For this review, take the finished solid that the model builds, in its own axes (mm). Face numbers are marked on the shaded views. Round coordinates to 2 decimals unless told otherwise and drop trailing zeros. Loops run counter-clockwise (first coordinate to the right, second up) from the corner with the lowest first, then second, coordinate; pieces in that order, holes last.
1. Clearance check with flat-ended pins moving along their axes: pin 1 Ø7.5 at (x, y) = (-84.5, 78.5) entering from +Z; pin 2 Ø2.5 at (y, z) = (-84.5, 11) entering from +X; pin 3 Ø4 at (x, z) = (-86.5, 10) entering from -Y. State where each tip first meets the part, or that it passes through.
2. Draft analysis for pull direction Y (two halves, no side actions). For the marked faces 1, 2, 3 and 4, state which applies: released by +Y, released by -Y, zero draft, split by the parting line, or undercut.
3. To check wall thickness, follow line 1 along Y through (x, z) = (-79.2, 12); line 2 along Y through (x, z) = (45, 9.5). State the ranges of each line that lie inside material, in increasing order.
4. Consider section A-A on x = -7.5. State the section outline as (y, z) points, then the cut area to 3 significant figures.
5. Consider section C-C on y = 85. State the section outline as (x, z) points, then the cut area to 3 significant figures.
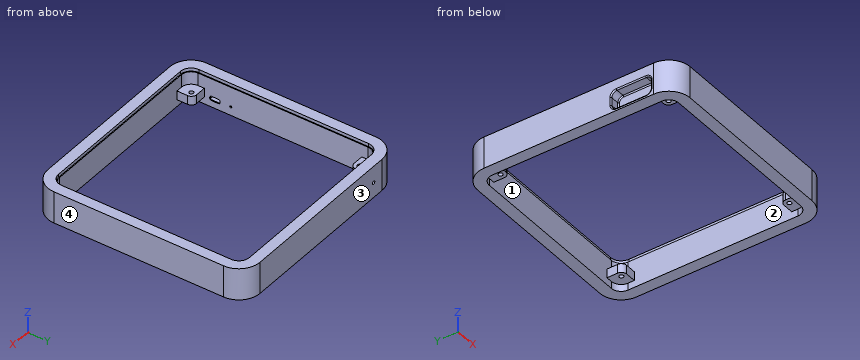
from build123d import *

# Parameters (mm, degrees)
SKETCH2_W                = 200
SKETCH2_H                = 200
BOSS_EXTRUDE1_DEPTH      = 30
FILLET1_R                = 20
CUT_EXTRUDE1_DEPTH       = 3
CUT_EXTRUDE2_DEPTH       = 28
SKETCH6_W                = 15
SKETCH6_H                = 15
BOSS_EXTRUDE4_DEPTH      = 15
FILLET2_R                = 5
F_4_0_4_DIAMETER_HOLE1_D = 4
CUT_EXTRUDE3_DEPTH       = 6.6
CUT_EXTRUDE4_REACH       = 202
SKETCH11_R               = 1.5
SKETCH15_R               = 1
CUT_EXTRUDE5_DEPTH       = 11.8
CUT_EXTRUDE7_DEPTH       = 9.8
FILLET3_R                = 1


with BuildPart() as part:
    # Sketch2 → Boss-Extrude1 (new body)
    with BuildSketch(Plane.XY):
        Rectangle(SKETCH2_W, SKETCH2_H)
    extrude(amount=BOSS_EXTRUDE1_DEPTH)

    # Fillet1
    fillet1_edges = [part.edges().sort_by_distance(p)[0] for p in [
        (100, -100, 15),
        (-100, -100, 15),
        (-100, 100, 15),
        (100, 100, 15),
    ]]
    fillet(fillet1_edges, radius=FILLET1_R)

    # Sketch3 → Cut-Extrude1 (cut)
    with BuildSketch(Plane.XY.offset(30)):
        with BuildLine():
            Line((-90, 80), (-90, -80))
            ThreePointArc((-90, -80), (-87.071067812, -87.071067812), (-80, -90))
            Line((-80, -90), (80, -90))
            ThreePointArc((80, -90), (87.071067812, -87.071067812), (90, -80))
            Line((90, -80), (90, 80))
            ThreePointArc((90, 80), (87.071067812, 87.071067812), (80, 90))
            Line((80, 90), (-80, 90))
            ThreePointArc((-80, 90), (-87.071067812, 87.071067812), (-90, 80))
        make_face()
    extrude(amount=-CUT_EXTRUDE1_DEPTH, mode=Mode.SUBTRACT)

    # Sketch4 → Cut-Extrude2 (cut, through all)
    with BuildSketch(Plane.XY.offset(27)):
        with BuildLine():
            Line((-89.2, 80), (-89.2, -80))
            ThreePointArc((-89.2, -80), (-86.505382387, -86.505382387), (-80, -89.2))
            Line((-80, -89.2), (80, -89.2))
            ThreePointArc((80, -89.2), (86.505382387, -86.505382387), (89.2, -80))
            Line((89.2, -80), (89.2, 80))
            ThreePointArc((89.2, 80), (86.505382387, 86.505382387), (80, 89.2))
            Line((80, 89.2), (-80, 89.2))
            ThreePointArc((-80, 89.2), (-86.505382387, 86.505382387), (-89.2, 80))
        make_face()
    extrude(amount=-CUT_EXTRUDE2_DEPTH, mode=Mode.SUBTRACT)

    # Sketch6 → Boss-Extrude4 (add)
    with BuildSketch(Plane(origin=(0, 0, 0), x_dir=(-1, 0, 0), z_dir=(0, 0, -1))):
        with Locations((-81.7, -81.7)):
            Rectangle(SKETCH6_W, SKETCH6_H)
        with Locations((-81.7, 81.7)):
            Rectangle(SKETCH6_W, SKETCH6_H)
        with Locations((81.7, 81.7)):
            Rectangle(SKETCH6_W, SKETCH6_H)
        with Locations((81.7, -81.7)):
            Rectangle(SKETCH6_W, SKETCH6_H)
    extrude(amount=-BOSS_EXTRUDE4_DEPTH)

    # Fillet2
    fillet2_edges = [part.edges().sort_by_distance(p)[0] for p in [
        (74.2, 74.2, 7.5),
        (-74.2, 74.2, 7.5),
        (-74.2, -74.2, 7.5),
        (74.2, -74.2, 7.5),
    ]]
    fillet(fillet2_edges, radius=FILLET2_R)

    # Ø4.0 (4) Diameter Hole1 (through all)
    with Locations(Plane(origin=(0, 0, 0), x_dir=(-1, 0, 0), z_dir=(0, 0, -1))):
        with Locations((-79.2, 79.2), (79.2, 79.2), (-79.2, -79.2), (79.2, -79.2)):
            Hole(F_4_0_4_DIAMETER_HOLE1_D / 2)

    # Sketch10 → Cut-Extrude3 (cut)
    with BuildSketch(Plane(origin=(0, 0, 0), x_dir=(-1, 0, 0), z_dir=(0, 0, -1))):
        with BuildLine():
            Line((89.2, -80), (89.2, 80))
            ThreePointArc((89.2, 80), (86.505382387, 86.505382387), (80, 89.2))
            Line((80, 89.2), (-80, 89.2))
            ThreePointArc((-80, 89.2), (-86.505382387, 86.505382387), (-89.2, 80))
            Line((-89.2, 80), (-89.2, -80))
            ThreePointArc((-89.2, -80), (-86.505382387, -86.505382387), (-80, -89.2))
            Line((-80, -89.2), (80, -89.2))
            ThreePointArc((80, -89.2), (86.505382387, -86.505382387), (89.2, -80))
        make_face()
    extrude(amount=-CUT_EXTRUDE3_DEPTH, mode=Mode.SUBTRACT)

    # Sketch11 → Cut-Extrude4 (cut, up to next)
    with BuildSketch(Plane(origin=(0, 100, 0), x_dir=(1, 0, 0), z_dir=(0, 1, 0)), mode=Mode.PRIVATE) as cut_extrude4_sk1:
        with Locations((-68.95500318, -14.324851484)):
            Circle(SKETCH11_R)
    cut_extrude4_tool1 = extrude(cut_extrude4_sk1.sketch, amount=-CUT_EXTRUDE4_REACH, mode=Mode.PRIVATE) & part.part
    add(cut_extrude4_tool1.solids().sort_by_distance((-68.955003, 100, 14.324851))[0], mode=Mode.SUBTRACT)

    # Sketch15 → Cut-Extrude5 (cut, through all)
    with BuildSketch(Plane(origin=(-89.2, 0, 0), x_dir=(0, 0, -1), z_dir=(1, 0, 0))):
        with Locations((-8.179999988, -49.23845191)):
            Circle(SKETCH15_R)
        with BuildLine():
            Line((-6.1, -64.178451904), (-6.1, -64.148451912))
            Line((-6.1, -64.148451912), (-6.1, -60.988451904))
            ThreePointArc((-6.1, -60.988451904), (-6.237016841, -60.299621726), (-6.627207794, -59.715659698))
            ThreePointArc((-6.627207794, -59.715659698), (-7.211170067, -59.325468644), (-7.90000053, -59.188451904))
            Line((-7.90000053, -59.188451904), (-8.46, -59.188451904))
            ThreePointArc((-8.46, -59.188451904), (-9.148830178, -59.325468746), (-9.732792206, -59.715659698))
            ThreePointArc((-9.732792206, -59.715659698), (-10.122983159, -60.299621726), (-10.26, -60.988451904))
            Line((-10.26, -60.988451904), (-10.26, -67.338451904))
            ThreePointArc((-10.26, -67.338451904), (-10.122983159, -68.027282082), (-9.732792205, -68.611244109))
            ThreePointArc((-9.732792205, -68.611244109), (-9.148830178, -69.001435061), (-8.46, -69.138451901))
            Line((-8.46, -69.138451901), (-7.900000051, -69.138451901))
            ThreePointArc((-7.900000051, -69.138451901), (-7.211169847, -69.001435069), (-6.627207798, -68.611244107))
            ThreePointArc((-6.627207798, -68.611244107), (-6.237016846, -68.02728208), (-6.100000002, -67.338451904))
            Line((-6.100000002, -67.338451904), (-6.1, -64.178451904))
        make_face()
    extrude(amount=-CUT_EXTRUDE5_DEPTH, mode=Mode.SUBTRACT)

    # Sketch17 → Cut-Extrude7 (cut)
    with BuildSketch(Plane.ZY.offset(100)):
        with BuildLine():
            Line((15.061316978, -39.847521487), (7.5, -39.847521487))
            ThreePointArc((7.5, -39.847521487), (3.964466094, -41.311987581), (2.5, -44.847521487))
            Line((2.5, -44.847521487), (2.5, -72.5))
            ThreePointArc((2.5, -72.5), (3.964466094, -76.035533906), (7.5, -77.5))
            Line((7.5, -77.5), (15.061316978, -77.5))
            ThreePointArc((15.061316978, -77.5), (18.596850884, -76.035533906), (20.061316978, -72.5))
            Line((20.061316978, -72.5), (20.061316978, -44.847521487))
            ThreePointArc((20.061316978, -44.847521487), (18.596850884, -41.311987581), (15.061316978, -39.847521487))
        make_face()
    extrude(amount=-CUT_EXTRUDE7_DEPTH, mode=Mode.SUBTRACT)

    # Fillet3
    fillet3_edges = [part.edges().sort_by_distance(p)[0] for p in [
        (-100, -41.311987581, 3.964466094),
        (-100, -58.673760744, 2.5),
        (-100, -76.035533906, 3.964466094),
        (-100, -77.5, 11.280658489),
        (-100, -76.035533906, 18.596850884),
        (-100, -58.673760744, 20.061316978),
        (-100, -41.311987581, 18.596850884),
        (-100, -39.847521487, 11.280658489),
        (-90.2, -41.311987581, 3.964466094),
        (-90.2, -39.847521487, 11.280658489),
        (-90.2, -41.311987581, 18.596850884),
        (-90.2, -58.673760744, 20.061316978),
        (-90.2, -76.035533906, 18.596850884),
        (-90.2, -77.5, 11.280658489),
        (-90.2, -76.035533906, 3.964466094),
        (-90.2, -58.673760744, 2.5),
    ]]
    fillet(fillet3_edges, radius=FILLET3_R)


solid = part.part
Resolved:
1. pin 1: stops at z = 15
1. pin 2: stops at x = 99.73
1. pin 3: stops at y = -99.49
2. face 1: undercut
2. face 2: undercut
2. face 3: released by +Y
2. face 4: zero draft
3. line 1: y = -100 to -81.2, -77.2 to -74.2, 74.2 to 77.2, 81.2 to 100
3. line 2: y = -100 to -89.2, 89.2 to 100
4. outline: (-100, 0) - (-89.2, 0) - (-89.2, 27) - (-90, 27) - (-90, 30) - (-100, 30) - close; (89.2, 0) - (100, 0) - (100, 30) - (90, 30) - (90, 27) - (89.2, 27) - close
4. area: 643 mm2
5. outline: (-99.36, 0) - (-87.72, 0) - (-87.72, 6.6) - (-74.2, 6.6) - (-74.2, 15) - (-87.72, 15) - (-87.72, 27) - (-88.66, 27) - (-88.66, 30) - (-99.36, 30) - close; (74.2, 6.6) - (87.72, 6.6) - (87.72, 0) - (99.36, 0) - (99.36, 30) - (88.66, 30) - (88.66, 27) - (87.72, 27) - (87.72, 15) - (74.2, 15) - close
5. area: 920 mm2
